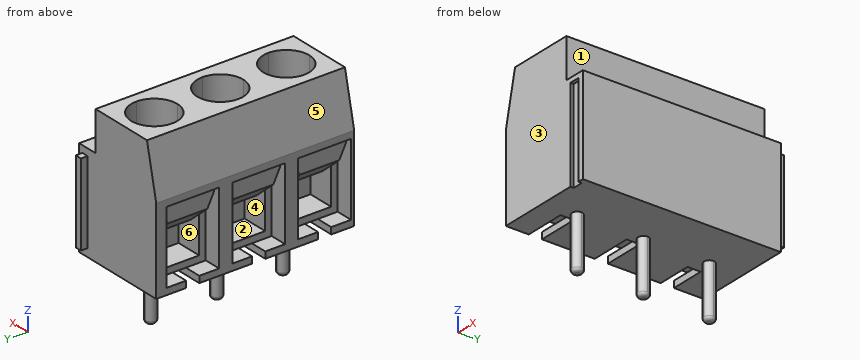
from build123d import *

# Parameters (mm, degrees)
F1_DEPTH  = 15
F3_DEPTH  = 3
F4_W      = 0.5
F4_H      = 0.5
F5_DEPTH  = 0.5
F6_DEPTH  = 1.3
F7_DEPTH  = 3.3
F8_SIZE   = 1
F9_W      = 0.7894294686
F9_H      = 7.0516658016
F10_DEPTH = 0.25
F11_W     = 0.5
F11_H     = 6.2580032973
F12_DEPTH = 0.5
F14_DEPTH = 4
F6_FACE_W = 1
F6_FACE_H = 0.5
F16_DEPTH = 2.6


# Not quite as in the source:
# - a fillet or chamfer that OpenCascade refuses, or shapes differently, is made with other operations: its cross-section is extruded or revolved along the edge and cut away or added


with BuildPart() as f1:
    # F0 (on Front) → F1 (new body)
    with BuildSketch(Plane.XZ):
        Polygon((-7.5, 0), (0, 0), (0, 7.397435054), (-1.6, 7.397435054), (-1.6, 10.397435054), (-6.6, 10.397435054), (-7.5, 6.5), align=None)
    extrude(amount=F1_DEPTH)

    # F2 (on face) → F3 (cut)
    with BuildSketch(Plane.XY.offset(10.397435054)):
        with BuildLine():
            ThreePointArc((-2.35, -2.5), (-2.8625631329, -1.2625631329), (-4.1, -0.75))
            Line((-4.1, -0.75), (-4.1, -2.5))
            Line((-4.1, -2.5), (-4.1, -4.25))
            ThreePointArc((-4.1, -4.25), (-2.8625631329, -3.7374368671), (-2.35, -2.5))
        make_face()
        with BuildLine():
            ThreePointArc((-2.35, -12.5), (-2.8625631329, -11.2625631329), (-4.1, -10.75))
            Line((-4.1, -10.75), (-4.1, -14.25))
            ThreePointArc((-4.1, -14.25), (-2.8625631329, -13.7374368671), (-2.35, -12.5))
        make_face()
        with BuildLine():
            Line((-4.1, -14.25), (-4.1, -10.75))
            ThreePointArc((-4.1, -10.75), (-5.85, -12.5), (-4.1, -14.25))
        make_face()
        with BuildLine():
            ThreePointArc((-2.35, -7.5), (-2.8625631329, -6.2625631329), (-4.1, -5.75))
            Line((-4.1, -5.75), (-4.1, -7.5))
            Line((-4.1, -7.5), (-2.35, -7.5))
        make_face()
        with BuildLine():
            Line((-4.1, -7.5), (-4.1, -5.75))
            ThreePointArc((-4.1, -5.75), (-5.85, -7.5), (-4.1, -9.25))
            Line((-4.1, -9.25), (-4.1, -7.5))
        make_face()
        with BuildLine():
            Line((-4.1, -2.5), (-4.1, -0.75))
            ThreePointArc((-4.1, -0.75), (-5.85, -2.5), (-4.1, -4.25))
            Line((-4.1, -4.25), (-4.1, -2.5))
        make_face()
        with BuildLine():
            Line((-2.35, -7.5), (-4.1, -7.5))
            Line((-4.1, -7.5), (-4.1, -9.25))
            ThreePointArc((-4.1, -9.25), (-2.8625631329, -8.7374368671), (-2.35, -7.5))
        make_face()
    extrude(amount=-F3_DEPTH, mode=Mode.SUBTRACT)

    # F4 (on face) → F5 (cut)
    with BuildSketch(Plane(origin=(-7.5, 0, 0), x_dir=(0, -1, 0), z_dir=(-1, 0, 0))):
        with Locations((2.510879118, 0.25)):
            Rectangle(F4_W, F4_H)
        with Locations((12.510879118, 0.25)):
            Rectangle(F4_W, F4_H)
        with Locations((7.510879118, 0.25)):
            Rectangle(F4_W, F4_H)
        with Locations((3.010879118, 0.25)):
            Rectangle(F4_W, F4_H)
        Polygon((0.760879118, 0.5), (2.260879118, 0.5), (2.760879118, 0.5), (2.760879118, 1), (1.260879118, 1), (1.260879118, 4.5), (0.760879118, 5.5), align=None)
        Polygon((2.760879118, 1), (2.760879118, 0.5), (3.260879118, 0.5), (4.760879118, 0.5), (4.760879118, 5.5), (4.260879118, 4.5), (4.260879118, 1), align=None)
        Polygon((0.760879118, 6), (0.760879118, 5.5), (1.260879118, 4.5), (1.760879118, 3.5), (2.760879118, 3.5), (2.760879118, 5.5), (2.760879118, 6), align=None)
        with Locations((8.010879118, 0.25)):
            Rectangle(F4_W, F4_H)
        Polygon((5.760879118, 0.5), (7.260879118, 0.5), (7.760879118, 0.5), (7.760879118, 1), (6.260879118, 1), (6.260879118, 4.5), (5.760879118, 5.5), align=None)
        Polygon((2.760879118, 5.5), (2.760879118, 3.5), (3.760879118, 3.5), (4.260879118, 4.5), (4.760879118, 5.5), (4.760879118, 6), (2.760879118, 6), align=None)
        Polygon((7.760879118, 1), (7.760879118, 0.5), (8.260879118, 0.5), (9.760879118, 0.5), (9.760879118, 5.5), (9.260879118, 4.5), (9.260879118, 1), align=None)
        Polygon((5.760879118, 6), (5.760879118, 5.5), (6.260879118, 4.5), (6.760879118, 3.5), (7.760879118, 3.5), (7.760879118, 5.5), (7.760879118, 6), align=None)
        with Locations((13.010879118, 0.25)):
            Rectangle(F4_W, F4_H)
        Polygon((10.760879118, 0.5), (12.260879118, 0.5), (12.760879118, 0.5), (12.760879118, 1), (11.260879118, 1), (11.260879118, 4.5), (10.760879118, 5.5), align=None)
        Polygon((7.760879118, 5.5), (7.760879118, 3.5), (8.760879118, 3.5), (9.260879118, 4.5), (9.760879118, 5.5), (9.760879118, 6), (7.760879118, 6), align=None)
        Polygon((12.760879118, 1), (12.760879118, 0.5), (13.260879118, 0.5), (14.760879118, 0.5), (14.760879118, 5.5), (14.260879118, 4.5), (14.260879118, 1), align=None)
        Polygon((10.760879118, 6), (10.760879118, 5.5), (11.260879118, 4.5), (11.760879118, 3.5), (12.760879118, 3.5), (12.760879118, 5.5), (12.760879118, 6), align=None)
        Polygon((12.760879118, 5.5), (12.760879118, 3.5), (13.760879118, 3.5), (14.260879118, 4.5), (14.760879118, 5.5), (14.760879118, 6), (12.760879118, 6), align=None)
        Polygon((1.260879118, 1), (2.760879118, 1), (2.760879118, 3.5), (1.760879118, 3.5), (1.260879118, 4.5), align=None)
        Polygon((2.760879118, 3.5), (2.760879118, 1), (4.260879118, 1), (4.260879118, 4.5), (3.760879118, 3.5), align=None)
        Polygon((6.260879118, 1), (7.760879118, 1), (7.760879118, 3.5), (6.760879118, 3.5), (6.260879118, 4.5), align=None)
        Polygon((7.760879118, 3.5), (7.760879118, 1), (9.260879118, 1), (9.260879118, 4.5), (8.760879118, 3.5), align=None)
        Polygon((11.260879118, 1), (12.760879118, 1), (12.760879118, 3.5), (11.760879118, 3.5), (11.260879118, 4.5), align=None)
        Polygon((12.760879118, 3.5), (12.760879118, 1), (14.260879118, 1), (14.260879118, 4.5), (13.760879118, 3.5), align=None)
    extrude(amount=-F5_DEPTH, mode=Mode.SUBTRACT)

    # F4 (on face) → F6 (cut)
    with BuildSketch(Plane(origin=(-7.5, 0, 0), x_dir=(0, -1, 0), z_dir=(-1, 0, 0))):
        Polygon((0.760879118, 0.5), (2.260879118, 0.5), (2.760879118, 0.5), (2.760879118, 1), (1.260879118, 1), (1.260879118, 4.5), (0.760879118, 5.5), align=None)
        Polygon((1.260879118, 1), (2.760879118, 1), (2.760879118, 3.5), (1.760879118, 3.5), (1.260879118, 4.5), align=None)
        Polygon((2.760879118, 3.5), (2.760879118, 1), (4.260879118, 1), (4.260879118, 4.5), (3.760879118, 3.5), align=None)
        Polygon((2.760879118, 1), (2.760879118, 0.5), (3.260879118, 0.5), (4.760879118, 0.5), (4.760879118, 5.5), (4.260879118, 4.5), (4.260879118, 1), align=None)
        Polygon((5.760879118, 0.5), (7.260879118, 0.5), (7.760879118, 0.5), (7.760879118, 1), (6.260879118, 1), (6.260879118, 4.5), (5.760879118, 5.5), align=None)
        Polygon((6.260879118, 1), (7.760879118, 1), (7.760879118, 3.5), (6.760879118, 3.5), (6.260879118, 4.5), align=None)
        Polygon((7.760879118, 3.5), (7.760879118, 1), (9.260879118, 1), (9.260879118, 4.5), (8.760879118, 3.5), align=None)
        Polygon((7.760879118, 1), (7.760879118, 0.5), (8.260879118, 0.5), (9.760879118, 0.5), (9.760879118, 5.5), (9.260879118, 4.5), (9.260879118, 1), align=None)
        Polygon((12.260879118, 0.5), (12.760879118, 0.5), (12.760879118, 1), (11.260879118, 1), (11.260879118, 4.5), (10.760879118, 5.5), (10.760879118, 0.5), align=None)
        Polygon((11.260879118, 1), (12.760879118, 1), (12.760879118, 3.5), (11.760879118, 3.5), (11.260879118, 4.5), align=None)
        Polygon((12.760879118, 3.5), (12.760879118, 1), (14.260879118, 1), (14.260879118, 4.5), (13.760879118, 3.5), align=None)
        Polygon((12.760879118, 0.5), (13.260879118, 0.5), (14.760879118, 0.5), (14.760879118, 5.5), (14.260879118, 4.5), (14.260879118, 1), (12.760879118, 1), align=None)
    extrude(amount=-F6_DEPTH, mode=Mode.SUBTRACT)

    # F4 (on face) → F7 (cut)
    with BuildSketch(Plane(origin=(-7.5, 0, 0), x_dir=(0, -1, 0), z_dir=(-1, 0, 0))):
        Polygon((1.260879118, 1), (2.760879118, 1), (2.760879118, 3.5), (1.760879118, 3.5), (1.260879118, 4.5), align=None)
        Polygon((2.760879118, 3.5), (2.760879118, 1), (4.260879118, 1), (4.260879118, 4.5), (3.760879118, 3.5), align=None)
        Polygon((6.260879118, 1), (7.760879118, 1), (7.760879118, 3.5), (6.760879118, 3.5), (6.260879118, 4.5), align=None)
        Polygon((7.760879118, 3.5), (7.760879118, 1), (9.260879118, 1), (9.260879118, 4.5), (8.760879118, 3.5), align=None)
        Polygon((11.260879118, 1), (12.760879118, 1), (12.760879118, 3.5), (11.760879118, 3.5), (11.260879118, 4.5), align=None)
        Polygon((12.760879118, 3.5), (12.760879118, 1), (14.260879118, 1), (14.260879118, 4.5), (13.760879118, 3.5), align=None)
    extrude(amount=-F7_DEPTH, mode=Mode.SUBTRACT)

    # F8
    f8_edges = [f1.edges().sort_by_distance(p)[0] for p in [
        (-7, -2.760879, 3.5),
        (-7, -7.760879, 3.5),
        (-7, -12.760879, 3.5),
    ]]
    chamfer(f8_edges, length=F8_SIZE)

    # F9 (on face) → F10 (cut)
    with BuildSketch(Plane.XZ.offset(15)):
        with Locations((-0.816616026, 3.5258329008)):
            Rectangle(F9_W, F9_H)
    extrude(amount=-F10_DEPTH, mode=Mode.SUBTRACT)

    # F11 (on face) → F12 (join)
    with BuildSketch(Plane(origin=(0, 0, 0), x_dir=(-1, 0, 0), z_dir=(0, 1, 0))):
        with Locations((0.5626286319, 3.7392643862)):
            Rectangle(F11_W, F11_H)
    extrude(amount=F12_DEPTH)

    # F13 (on face) → F14 (join)
    with BuildSketch(Plane(origin=(0, 0, 0), x_dir=(1, 0, 0), z_dir=(0, 0, -1))):
        with BuildLine():
            ThreePointArc((-3.35, 12.5), (-3.4671572875, 12.7828427125), (-3.75, 12.9))
            Line((-3.75, 12.9), (-3.75, 12.5))
            Line((-3.75, 12.5), (-3.75, 12.1))
            ThreePointArc((-3.75, 12.1), (-3.4671572875, 12.2171572875), (-3.35, 12.5))
        make_face()
        with BuildLine():
            ThreePointArc((-3.35, 2.5), (-3.4671572875, 2.7828427125), (-3.75, 2.9))
            Line((-3.75, 2.9), (-3.75, 2.1))
            ThreePointArc((-3.75, 2.1), (-3.4671572875, 2.2171572875), (-3.35, 2.5))
        make_face()
        with BuildLine():
            Line((-3.75, 2.1), (-3.75, 2.9))
            ThreePointArc((-3.75, 2.9), (-4.15, 2.5), (-3.75, 2.1))
        make_face()
        with BuildLine():
            ThreePointArc((-3.35, 7.5), (-3.4671572875, 7.7828427125), (-3.75, 7.9))
            Line((-3.75, 7.9), (-3.75, 7.5))
            Line((-3.75, 7.5), (-3.35, 7.5))
        make_face()
        with BuildLine():
            Line((-3.75, 7.5), (-3.75, 7.9))
            ThreePointArc((-3.75, 7.9), (-4.15, 7.5), (-3.75, 7.1))
            Line((-3.75, 7.1), (-3.75, 7.5))
        make_face()
        with BuildLine():
            Line((-3.75, 12.5), (-3.75, 12.9))
            ThreePointArc((-3.75, 12.9), (-4.15, 12.5), (-3.75, 12.1))
            Line((-3.75, 12.1), (-3.75, 12.5))
        make_face()
        with BuildLine():
            Line((-3.35, 7.5), (-3.75, 7.5))
            Line((-3.75, 7.5), (-3.75, 7.1))
            ThreePointArc((-3.75, 7.1), (-3.4671572875, 7.2171572875), (-3.35, 7.5))
        make_face()
    extrude(amount=F14_DEPTH)

    # F15: fillet of radius 0.25 on 3 edges, made by hand

    # F15_s1 → F15_t2 (revolve, cut)
    with BuildSketch(Plane.YZ.offset(-3.75)):
        with BuildLine():
            ThreePointArc((-12.9, -3.75), (-12.8267766953, -3.9267766953), (-12.65, -4))
            Line((-12.65, -4), (-12.9, -4))
            Line((-12.9, -4), (-12.9, -3.75))
        make_face()
    revolve(axis=Axis((-3.75, -12.5, -4), (0, 0, -1)), mode=Mode.SUBTRACT)

    # F15_s3 → F15_t4 (revolve, cut)
    with BuildSketch(Plane.YZ.offset(-3.75)):
        with BuildLine():
            ThreePointArc((-7.1, -3.75), (-7.1732233047, -3.9267766953), (-7.35, -4))
            Line((-7.35, -4), (-7.1, -4))
            Line((-7.1, -4), (-7.1, -3.75))
        make_face()
    revolve(axis=Axis((-3.75, -7.5, -4), (0, 0, -1)), mode=Mode.SUBTRACT)

    # F15_s5 → F15_t6 (revolve, cut)
    with BuildSketch(Plane.YZ.offset(-3.75)):
        with BuildLine():
            ThreePointArc((-2.9, -3.75), (-2.8267766953, -3.9267766953), (-2.65, -4))
            Line((-2.65, -4), (-2.9, -4))
            Line((-2.9, -4), (-2.9, -3.75))
        make_face()
    revolve(axis=Axis((-3.75, -2.5, -4), (0, 0, -1)), mode=Mode.SUBTRACT)

    # F6_face (on face) + F4 (on face) → F16 (cut)
    with BuildSketch(Plane(origin=(-7, -12.760879118, 0.25), x_dir=(0, -1, 0), z_dir=(-1, 0, 0))):
        Rectangle(F6_FACE_W, F6_FACE_H)
        with Locations((-5, 0)):
            Rectangle(F6_FACE_W, F6_FACE_H)
    with BuildSketch(Plane(origin=(-7.5, 0, 0), x_dir=(0, -1, 0), z_dir=(-1, 0, 0))):
        with Locations((3.010879118, 0.25)):
            Rectangle(F4_W, F4_H)
        with Locations((2.510879118, 0.25)):
            Rectangle(F4_W, F4_H)
    extrude(amount=-F16_DEPTH, mode=Mode.SUBTRACT)


solid = f1.part
Verification items for the finished model (mm, model axes). Face numbers are marked on the shaded views. A direction names the side the tool comes from. Give positions to 0.01 mm unless a question says otherwise; leave off trailing zeros. Loops run counter-clockwise (first coordinate to the right, second up) from the corner with the lowest first, then second, coordinate; pieces in that order, holes last.
1) Thickness scan on line 1 along Y through (x, z) = (-4.25, 9.5); line 2 along Y through (x, z) = (-3.75, -3.25); line 3 along X through (y, z) = (-7.25, 2.75). Record the ranges inside material, lowest first.
2) Depth check by flat-ended pin: pin 1 Ø1 at (x, z) = (-5.5, 2.5) entering from +Y; pin 2 Ø3 at (x, y) = (-4, -12.5) entering from +Z; pin 3 Ø1.5 at (y, z) = (-5.5, -1.5) entering from -X; pin 4 Ø0.9 at (y, z) = (-13, 2.5) entering from -X. Enter the tip coordinate at first touch or a pass-through.
3) Sectioned sample at D-D, the plane y = -9. Enter the section's corners in (x, z).
4) Sectioned sample at C-C, the plane z = 9.75. Enter the section's corners in (x, y).
5) Set-up check for the marked faces 5 and 6: record each of +Z, -Z, +X, -X, +Y, -Y from which the full face is reachable in a straight line by a thin tool's end or side.
6) Sectioned sample at A-A, the plane z = 5.75. Enter the section's corners in (x, y).
7) Sectioned sample at B-B, the plane z = -1. Enter the section's corners in (x, y).
8) Draft check along Y on the marked faces 1, 2, 3 and 4. Enter one of: pulls with the +Y half, pulls with the -Y half, needs draft (parallel to the pull), parting line crosses it, or undercut.
Answers:
1. line 1: y = -15 to -14.24, -10.76 to -9.24, -5.76 to -4.24, -0.76 to 0
1. line 2: y = -12.9 to -12.1, -7.9 to -7.1, -2.9 to -2.1
1. line 3: x = -4.2 to 0
2. pin 1: stops at y = 0
2. pin 2: stops at z = 7.4
2. pin 3: passes through
2. pin 4: stops at x = -4.2
3. outline: (-7.5, 0) - (0, 0) - (0, 7.4) - (-1.6, 7.4) - (-1.6, 10.4) - (-3.2, 10.4) - (-3.2, 7.4) - (-5, 7.4) - (-5, 10.4) - (-6.6, 10.4) - (-7.5, 6.5) - (-7.5, 6) - (-7, 6) - (-7, 4.5) - (-6.48, 3.98) - (-4.2, 3.98) - (-4.2, 1) - (-6.2, 1) - (-6.2, 0.5) - (-7.5, 0.5) - close
4. outline: (-6.75, -15) - (-1.6, -15) - (-1.6, 0) - (-6.75, 0) - close; hole circle Ø3.5 at (-4.1, -12.5); hole circle Ø3.5 at (-4.1, -7.5); hole circle Ø3.5 at (-4.1, -2.5)
5. face 5: +Z, -X, +Y, -Y
5. face 6: -X
6. outline: (-7.5, -15) - (-1.21, -15) - (-1.21, -14.75) - (-0.42, -14.75) - (-0.42, -15) - (0, -15) - (0, 0) - (-0.31, 0) - (-0.31, 0.5) - (-0.81, 0.5) - (-0.81, 0) - (-7.5, 0) - (-7.5, -0.76) - (-7, -0.76) - (-7, -4.76) - (-7.5, -4.76) - (-7.5, -5.76) - (-7, -5.76) - (-7, -9.76) - (-7.5, -9.76) - (-7.5, -10.76) - (-7, -10.76) - (-7, -14.76) - (-7.5, -14.76) - close
7. outline: circle Ø0.8 at (-3.75, -12.5); circle Ø0.8 at (-3.75, -7.5); circle Ø0.8 at (-3.75, -2.5)
8. face 1: needs draft
8. face 2: undercut
8. face 3: pulls with the -Y half
8. face 4: undercut
